from build123d import *

# Parameters (mm, degrees)
SKETCH_11_W              = 120
SKETCH_11_H              = 80
EXTRUDE_3_DEPTH          = 80
EXTRUDE_3_TAPER          = 14
CUT_EXTRUDE_START        = 80
SKETCH_12_W              = 40
SKETCH_12_H              = 5
CUT_EXTRUDE_1_DEPTH      = 20
CUT_EXTRUDE_2_DEPTH      = 108.70329631
CUT_EXTRUDE_2_DEPTH_BACK = 108.70329631
SKETCH_13_R              = 30


with BuildPart() as part:
    # 스케치11 → 보스-돌출3 (new body)
    with BuildSketch(Plane(origin=(0, 0, 0), x_dir=(1, 0, 0), z_dir=(0, 1, 0))):
        Rectangle(SKETCH_11_W, SKETCH_11_H)
    extrude(amount=EXTRUDE_3_DEPTH, taper=EXTRUDE_3_TAPER)

    # 스케치12 → 컷-돌출1 (cut)
    with BuildSketch(Plane(origin=(0, 0, 0), x_dir=(1, 0, 0), z_dir=(0, 1, 0)).offset(CUT_EXTRUDE_START)):
        Rectangle(SKETCH_12_W, SKETCH_12_H)
    extrude(amount=-CUT_EXTRUDE_1_DEPTH, mode=Mode.SUBTRACT)

    # 스케치13 → 컷-돌출2 (cut, two sides: drawn at the far end of the back side and taken through both)
    with BuildSketch(Plane.XY.offset(-CUT_EXTRUDE_2_DEPTH_BACK)):
        Circle(SKETCH_13_R)
    extrude(amount=CUT_EXTRUDE_2_DEPTH + CUT_EXTRUDE_2_DEPTH_BACK, mode=Mode.SUBTRACT)


solid = part.part
For this review, take the finished solid that the model builds, in its own axes (mm). A direction names the side the tool comes from. Round coordinates to 2 decimals unless told otherwise and drop trailing zeros. Write each question's results on one line, items separated by ' | '. Start each with the question number.
1. Clearance check with flat-ended pins moving along their axes: pin 1 Ø22 at (x, y) = (6.5, 68) entering from +Z; pin 2 Ø5.5 at (y, z) = (68, 1) entering from -X; pin 3 Ø3 at (y, z) = (35.5, 19.5) entering from +X. State where each tip first meets the part, or that it passes through.
2. Draft analysis for pull direction Z (two halves, no side actions). For faces 3 (the face through (-20, 70, 0)), 4 (the face through (44, 0, 0)), state which applies: pulls with the +Z half, pulls with the -Z half, needs draft (parallel to the pull), parting line crosses it, or undercut.
3. Tool access review of faces 1 (the face through (0, 60, 0)), 2 (the face through (3, 80, 7)): name each direction out of +Z, -Z, +X, -X, +Y, -Y from which nothing blocks a thin tool from reaching the whole face with its end or side.
4. To check wall thickness, follow L1, parallel to Z at x = -16.5, y = 68; L2, parallel to X at y = 8.5, z = 18; L3, parallel to Z at x = -13, y = 64.5. State the ranges of each line that lie inside material, in increasing order. Write a range as [from, to].
Output values:
1) pin 1: z = 25.79 | pin 2: x = -43.73 | pin 3: x = 51.52
2) face 3: undercut | face 4: needs draft
3) face 1: +Y | face 2: +Z, -Z, +X, -X, +Y
4) L1: [-23.05, -2.5], [2.5, 23.05] | L2: [-57.88, -28.77], [28.77, 57.88] | L3: [-23.92, -2.5], [2.5, 23.92]
